from build123d import *

# Parameters (mm, degrees)
F0_W         = 50.8
F0_H         = 38.1
F1_DEPTH     = 50.8
F2_T2_ANGLE  = 53.6002837339
F2_T4_ANGLE  = 53.6002837339
F2_T6_ANGLE  = 109.3939294159
F2_T8_ANGLE  = 109.3939294159
F2_T10_ANGLE = 342.5650608066
F2_T12_ANGLE = 342.5650608066
F2_T14_ANGLE = 359.64
F2_T16_ANGLE = 359.64


# Not quite as in the source:
# - a fillet or chamfer that OpenCascade refuses, or shapes differently, is made with other operations: its cross-section is extruded or revolved along the edge and cut away or added


with BuildPart() as f1:
    # F0 (on Front) → F1 (new body)
    with BuildSketch(Plane.XZ):
        with BuildLine():
            Line((-177.8, 0), (0, 0))
            Line((0, 0), (0, -76.2))
            Line((0, -76.2), (127, -76.2))
            ThreePointArc((127, -76.2), (137.069140052, -63.7754848813), (151.3100119581, -71.0524158741))
            ThreePointArc((151.3100119581, -71.0524158741), (163.8205179064, -114.6223435958), (164.0100119581, -159.9524158741))
            Line((164.0100119581, -159.9524158741), (213.1969004549, -147.2524158741))
            ThreePointArc((213.1969004549, -147.2524158741), (216.0088779453, -71.4162966266), (170.7058872965, -10.53392448))
            ThreePointArc((170.7058872965, -10.53392448), (166.5887281869, -5.9663543586), (165.1, 0))
            ThreePointArc((165.1, 0), (161.3802561211, 8.9802561211), (152.4, 12.7))
            Line((152.4, 12.7), (152.4, 50.8))
            Line((152.4, 50.8), (-177.8, 50.8))
            Line((-177.8, 50.8), (-177.8, 0))
        make_face()
        with Locations((98.425, -53.975)):
            Rectangle(F0_W, F0_H, mode=Mode.SUBTRACT)
    extrude(amount=F1_DEPTH)

    # F2: fillet of radius 25.4 on 8 edges, made by hand

    # F2_s1 → F2_t2 (revolve, cut)
    with BuildSketch(Plane(origin=(51.1854271814, 0, -115.4451111674), x_dir=(0, 1, 0), z_dir=(-0.4053215847, 0, 0.9141741699))):
        with BuildLine():
            ThreePointArc((-25.4, -109.5246267837), (-43.3605122421, -116.9641145416), (-50.8, -134.9246267837))
            Line((-50.8, -134.9246267837), (-50.8, -109.5246267837))
            Line((-50.8, -109.5246267837), (-25.4, -109.5246267837))
        make_face()
    revolve(axis=Axis((0.3798565029, -50.8, -137.9710095106), (0, 1, 0)), revolution_arc=F2_T2_ANGLE, mode=Mode.SUBTRACT)

    # F2_s3 → F2_t4 (revolve, cut)
    with BuildSketch(Plane(origin=(51.1854271814, 0, -115.4451111674), x_dir=(0, 1, 0), z_dir=(-0.4053215847, 0, 0.9141741699))):
        with BuildLine():
            ThreePointArc((-25.4, -109.5246267837), (-7.4394877579, -116.9641145416), (0, -134.9246267837))
            Line((0, -134.9246267837), (0, -109.5246267837))
            Line((0, -109.5246267837), (-25.4, -109.5246267837))
        make_face()
    revolve(axis=Axis((0.3798565029, 0, -137.9710095106), (0, 1, 0)), revolution_arc=F2_T4_ANGLE, mode=Mode.SUBTRACT)

    # F2_s5 → F2_t6 (revolve, cut)
    with BuildSketch(Plane(origin=(18.3403057366, 0, 13.6443784603), x_dir=(0, 1, 0), z_dir=(-0.802321654, 0, -0.5968919194))):
        with BuildLine():
            ThreePointArc((-25.4, 262.599154914), (-43.3605122421, 255.1596671561), (-50.8, 237.199154914))
            Line((-50.8, 237.199154914), (-50.8, 262.599154914))
            Line((-50.8, 262.599154914), (-25.4, 262.599154914))
        make_face()
    revolve(axis=Axis((106.8588729648, -50.8, -105.3392447997), (0, -1, 0)), revolution_arc=F2_T6_ANGLE, mode=Mode.SUBTRACT)

    # F2_s7 → F2_t8 (revolve, cut)
    with BuildSketch(Plane(origin=(18.3403057366, 0, 13.6443784603), x_dir=(0, 1, 0), z_dir=(-0.802321654, 0, -0.5968919194))):
        with BuildLine():
            ThreePointArc((-25.4, 262.599154914), (-7.4394877579, 255.1596671561), (0, 237.199154914))
            Line((0, 237.199154914), (0, 262.599154914))
            Line((0, 262.599154914), (-25.4, 262.599154914))
        make_face()
    revolve(axis=Axis((106.8588729648, 0, -105.3392447997), (0, -1, 0)), revolution_arc=F2_T8_ANGLE, mode=Mode.SUBTRACT)

    # F2_s9 → F2_t10 (revolve, cut)
    with BuildSketch(Plane(origin=(122.3220401021, 0, -82.378257055), x_dir=(0, 1, 0), z_dir=(0.8294428724, 0, -0.5585915515))):
        with BuildLine():
            ThreePointArc((-25.4, 86.6175778493), (-7.4394877579, 79.1780900914), (0, 61.2175778493))
            Line((0, 61.2175778493), (0, 86.6175778493))
            Line((0, 86.6175778493), (-25.4, 86.6175778493))
        make_face()
    revolve(axis=Axis((177.8, 0, 0), (0, 1, 0)), revolution_arc=F2_T10_ANGLE, mode=Mode.SUBTRACT)

    # F2_s11 → F2_t12 (revolve, cut)
    with BuildSketch(Plane(origin=(122.3220401021, 0, -82.378257055), x_dir=(0, 1, 0), z_dir=(0.8294428724, 0, -0.5585915515))):
        with BuildLine():
            ThreePointArc((-25.4, 86.6175778493), (-43.3605122421, 79.1780900914), (-50.8, 61.2175778493))
            Line((-50.8, 61.2175778493), (-50.8, 86.6175778493))
            Line((-50.8, 86.6175778493), (-25.4, 86.6175778493))
        make_face()
    revolve(axis=Axis((177.8, -50.8, 0), (0, 1, 0)), revolution_arc=F2_T12_ANGLE, mode=Mode.SUBTRACT)

    # F2_s13 → F2_t14 (revolve, cut)
    with BuildSketch(Plane(origin=(50.2149791059, 0, -115.2044645561), x_dir=(0, 1, 0), z_dir=(-0.3995696961, 0, 0.9167028188))):
        with BuildLine():
            ThreePointArc((-25.4, -110.3161729414), (-7.4394877579, -117.7556606993), (0, -135.7161729414))
            Line((0, -135.7161729414), (0, -110.3161729414))
            Line((0, -110.3161729414), (-25.4, -110.3161729414))
        make_face()
    revolve(axis=Axis((139.7, 0, -76.2), (0, 1, 0)), revolution_arc=F2_T14_ANGLE, mode=Mode.SUBTRACT)

    # F2_s15 → F2_t16 (revolve, cut)
    with BuildSketch(Plane(origin=(50.2149791059, 0, -115.2044645561), x_dir=(0, 1, 0), z_dir=(-0.3995696961, 0, 0.9167028188))):
        with BuildLine():
            ThreePointArc((-25.4, -110.3161729414), (-43.3605122421, -117.7556606993), (-50.8, -135.7161729414))
            Line((-50.8, -135.7161729414), (-50.8, -110.3161729414))
            Line((-50.8, -110.3161729414), (-25.4, -110.3161729414))
        make_face()
    revolve(axis=Axis((139.7, -50.8, -76.2), (0, 1, 0)), revolution_arc=F2_T16_ANGLE, mode=Mode.SUBTRACT)


solid = f1.part
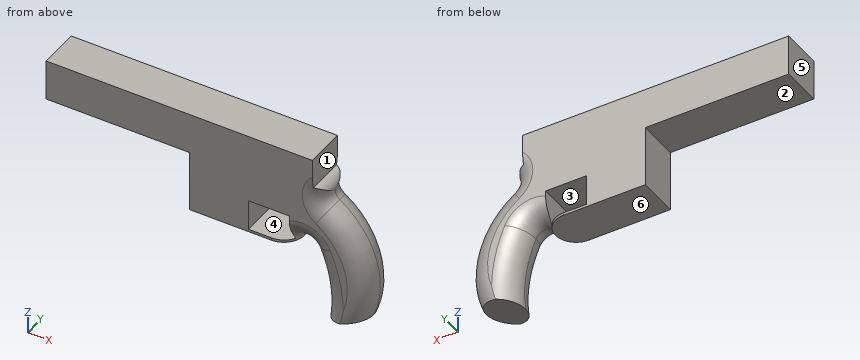
Read the model definition and answer for the solid it produces. Units are mm, in the model's axes. Face numbers are marked on the shaded views. A direction names the side the tool comes from. Coordinates: 2 decimals unless noted, no trailing zeros. Write each loop counter-clockwise with the first axis right and the second up, starting at its lowest first coordinate (ties: lowest second). Pieces come first, ordered by that corner, then holes. Notation, with made-up numbers: (52, 85) -> (97, 85) arc R6 ccw to (97, 91) -> close; hole circle Ø1 at (11, 39.5). An arc over 180 degrees is marked (long way). Return JSON: item names as keys, results as strings.
(1) The part is cut by section A-A on y = -45. Give the vertices of the cut face in (x, z) (1 decimal), then the cut area to 3 significant figures.
Answers below:
{"outline": "(-177.8, 0) -> (0, 0) -> (0, -76.2) -> (117.8, -76.2) arc R21.9 cw to (118, -73) -> (73, -73) -> (73, -34.9) -> (123.8, -34.9) -> (123.8, -61) arc R21.9 cw to (159.8, -67.3) arc R174.3 cw to (173.6, -157.5) -> (201.9, -150.2) arc R105.1 ccw to (165.5, -18.2) arc R21.9 cw to (158.8, 11) arc R12.7 ccw to (152.4, 12.7) -> (152.4, 50.8) -> (-177.8, 50.8) -> close", "area": "31,100 mm^2"}
(2) The part is cut by section D-D on z = -65. State how many separate pieces and enclosed holes the cut face has, then the cut area to 3 significant figures.
Answers below:
{"separate pieces": "3", "enclosed holes": "0", "area": "6,700 mm^2"}
(3) Each of these flat-tipped pins is pushed along its axis until it touches: P1, Ø15, axis at x = -96.5, y = -34, coming from the -Z side; P2, Ø1.5, axis at x = 82.5, y = -45.5, coming from the -Z side; P3, Ø11.5, axis at y = -33.5, z = -56, coming from the -X side. Where does it stop, or does it pass through?
Answers below:
{"P1": "z = 0", "P2": "z = -76.2", "P3": "x = 0"}
(4) Consider line 1 along Z through (x, y) = (108, -48) (3 decimals); line 2 along X through (y, z) = (-6.5, 29.5); line 3 along Z through (x, y) = (-115.5, -38). Determine where each line is inside the solid, lowest interval first. Write a range as from..to.
Answers below:
{"line 1": "-76.2..-73.025, -34.925..50.8", "line 2": "-177.8..152.4", "line 3": "0..50.8"}
(5) Which of the six approach directions +Z, -Z, +X, -X, +Y, -Y give full straight-line access (tool end or side, diameter ignored) to the marked faces 1, 2 and 3?
Answers below:
{"face 1": "+Z, +X, +Y, -Y", "face 2": "-Z, -X, +Y, -Y", "face 3": "+Y, -Y"}
(6) For a pull along X with two mould halves and no side action, classify the marked faces 4, 5 and 6 as pulls with the +X half, pulls with the -X half, needs draft (parallel to the pull), parting line crosses it, or undercut.
Answers below:
{"face 4": "undercut", "face 5": "pulls with the -X half", "face 6": "needs draft"}
(7) The part is cut by section C-C on y = -20. Give the vertices of the cut face in (x, z) (3 decimals), then the cut area to 3 significant figures.
Answers below:
{"outline": "(-177.8, 0) -> (0, 0) -> (0, -76.2) -> (126.419, -76.2) arc R13.281 cw to (151.841, -70.817) arc R165.681 cw to (164.617, -159.796) -> (212.501, -147.432) arc R113.719 ccw to (170.382, -11.016) arc R13.281 cw to (164.803, 2.73) arc R12.7 ccw to (152.4, 12.7) -> (152.4, 50.8) -> (-177.8, 50.8) -> close; hole (73.025, -73.025) -> (123.825, -73.025) -> (123.825, -34.925) -> (73.025, -34.925) -> close", "area": "33,800 mm^2"}
(8) The part is cut by section B-B on x = 52. Give the vertices of the cut face in (y, z).
Answers below:
{"outline": "(-50.8, -76.2) -> (0, -76.2) -> (0, 50.8) -> (-50.8, 50.8) -> close"}
